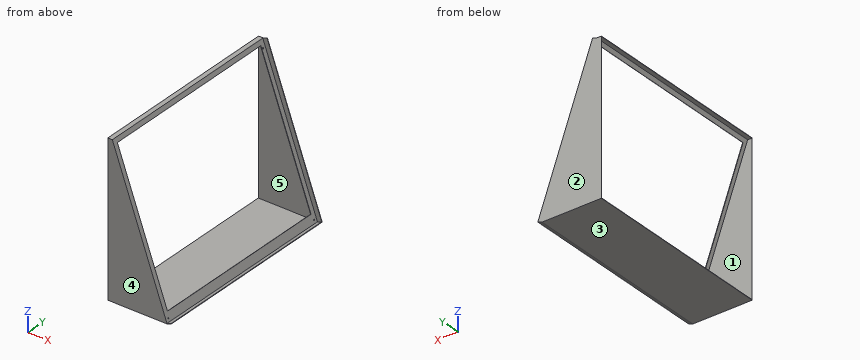
from build123d import *

# Parameters (mm, degrees)
F1_DEPTH = 650
F2_T     = -3
F3_W     = 1237
F3_H     = 974.1777724759
F4_DEPTH = 3
F5_W     = 3
F5_H     = 1061.1777724759
F6_DEPTH = 30
F7_R     = 4
F8_DEPTH = 25


with BuildPart() as f1:
    # F0 (on Front) → F1 (new body, symmetric)
    with BuildSketch(Plane.XZ):
        Polygon((-393.9702342662, 0), (0, 0), (28.1907786236, 10.2606042998), (27.1647181936, 13.0796821621), (-1.02606043, 2.8190778624), (-363.9702342662, 1000), (-393.9702342662, 1000), align=None)
    extrude(amount=F1_DEPTH, both=True)

    # F2
    f2_openings = [f1.faces().sort_by_distance(p)[0] for p in [
        (-393.970234, 0, 500),
    ]]
    offset(amount=F2_T, openings=f2_openings)

    # F3 (on face) → F4 (cut)
    with BuildSketch(Plane(origin=(0, 0, 0), x_dir=(0, 1, 0), z_dir=(0.9396926208, 0, 0.3420201433))):
        with Locations((-1.5, 547.088886238)):
            Rectangle(F3_W, F3_H)
    extrude(amount=-F4_DEPTH, mode=Mode.SUBTRACT)

    # F5 (on face) → F6 (join)
    with BuildSketch(Plane(origin=(0, 0, 0), x_dir=(0, 1, 0), z_dir=(0.9396926208, 0, 0.3420201433))):
        with Locations((648.5, 533.588886238)):
            Rectangle(F5_W, F5_H)
    extrude(amount=F6_DEPTH)

    # F7 (on face) → F8 (cut)
    with BuildSketch(Plane(origin=(0, 0, 0), x_dir=(0, 1, 0), z_dir=(0.9396926208, 0, 0.3420201433))):
        with Locations((627, 23)):
            Circle(F7_R)
        with Locations((-630, 23)):
            Circle(F7_R)
        with Locations((627, 1014.1777724759)):
            Circle(F7_R)
    extrude(amount=-F8_DEPTH, mode=Mode.SUBTRACT)


solid = f1.part
For this review, take the finished solid that the model builds, in its own axes (mm). Face numbers are marked on the shaded views. A direction names the side the tool comes from. Round coordinates to 2 decimals unless told otherwise and drop trailing zeros. Loops run counter-clockwise (first coordinate to the right, second up) from the corner with the lowest first, then second, coordinate; pieces in that order, holes last. Notation, with made-up numbers: (3.5, 33.5) - (31.5, 33.5) arc R7 cw to (31.5, 46.5) - close; hole circle Ø4 at (9, -3.75). An arc over 180 degrees is marked (long way). Answer as CSV lines item,"result".
(1) Consider section B-B on z = 519. Give the boundary of the cut face in (x, y).
Checked values:
outline,"(-393.97, -650) - (-188.9, -650) - (-188.9, -620) - (-192.09, -620) - (-192.09, -647) - (-393.97, -647) - close; (-393.97, 647) - (-192.09, 647) - (-192.09, 617) - (-188.9, 617) - (-188.9, 647) - (-156.98, 647) - (-156.98, 650) - (-393.97, 650) - close"
(2) Tool access review of the marked faces 4 and 5: name each direction out of +Z, -Z, +X, -X, +Y, -Y from which nothing blocks a thin tool from reaching the whole face with its end or side.
Checked values:
face 4,"+Z, -Z, +X, -X, -Y"
face 5,"-X"
(3) Insertion check: P1, Ø12, axis at x = -283.5, y = 388, coming from the -Z side; P2, Ø3, axis at x = -166.5, y = 287, coming from the +Z side; P3, Ø9, axis at x = -373.5, y = -133, coming from the +Z side. Each pin has a flat end and moves straight along its axis. Give the tip position at first contact, or say it passes through.
Checked values:
P1,"stops at z = 0"
P2,"stops at z = 3"
P3,"stops at z = 1000"
(4) Consider section D-D on z = 312.5. Give the boundary of the cut face in (x, y).
Checked values:
outline,"(-393.97, -650) - (-113.74, -650) - (-113.74, -620) - (-116.93, -620) - (-116.93, -647) - (-393.97, -647) - close; (-393.97, 647) - (-116.93, 647) - (-116.93, 617) - (-113.74, 617) - (-113.74, 647) - (-81.82, 647) - (-81.82, 650) - (-393.97, 650) - close"
(5) Consider section A-A on y = 541. Give the boundary of the cut face in (x, z), then the cut area to 3 significant figures.
Checked values:
outline,"(-393.97, 0) - (0, 0) - (28.19, 10.26) - (27.16, 13.08) - (-1.03, 2.82) - (-20.52, 56.38) - (-23.34, 55.36) - (-4.28, 3) - (-393.97, 3) - close; (-393.97, 997) - (-366.07, 997) - (-356.53, 970.78) - (-353.71, 971.81) - (-363.97, 1000) - (-393.97, 1000) - close"
area,"1,610 mm2"
(6) Mouldability with a two-part tool opening along Y and no side actions: class the marked faces 1, 2 and 3 as +Y half, -Y half, draft (parallel to the pull), parting line (faces both ways), or undercut.
Checked values:
face 1,"undercut"
face 2,"+Y half"
face 3,"draft"
(7) Consider section C-C on x = -306.5. Give the boundary of the cut face in (y, z).
Checked values:
outline,"(-650, 0) - (650, 0) - (650, 929.82) - (647, 929.82) - (647, 842.1) - (617, 842.1) - (617, 833.33) - (647, 833.33) - (647, 3) - (-647, 3) - (-647, 833.33) - (-620, 833.33) - (-620, 842.1) - (-650, 842.1) - close"
(8) Wall thickness on line 1 (Y direction, x = -238, z = 329.5); line 2 (Y direction, x = -299, z = 845); line 3 (Z direction, x = -231.5, y = -169): over which ranges is each line inside the solid? List them lowest first.
Checked values:
line 1,"y = -650 to -647, 647 to 650"
line 2,"y = 647 to 650"
line 3,"z = 0 to 3"
